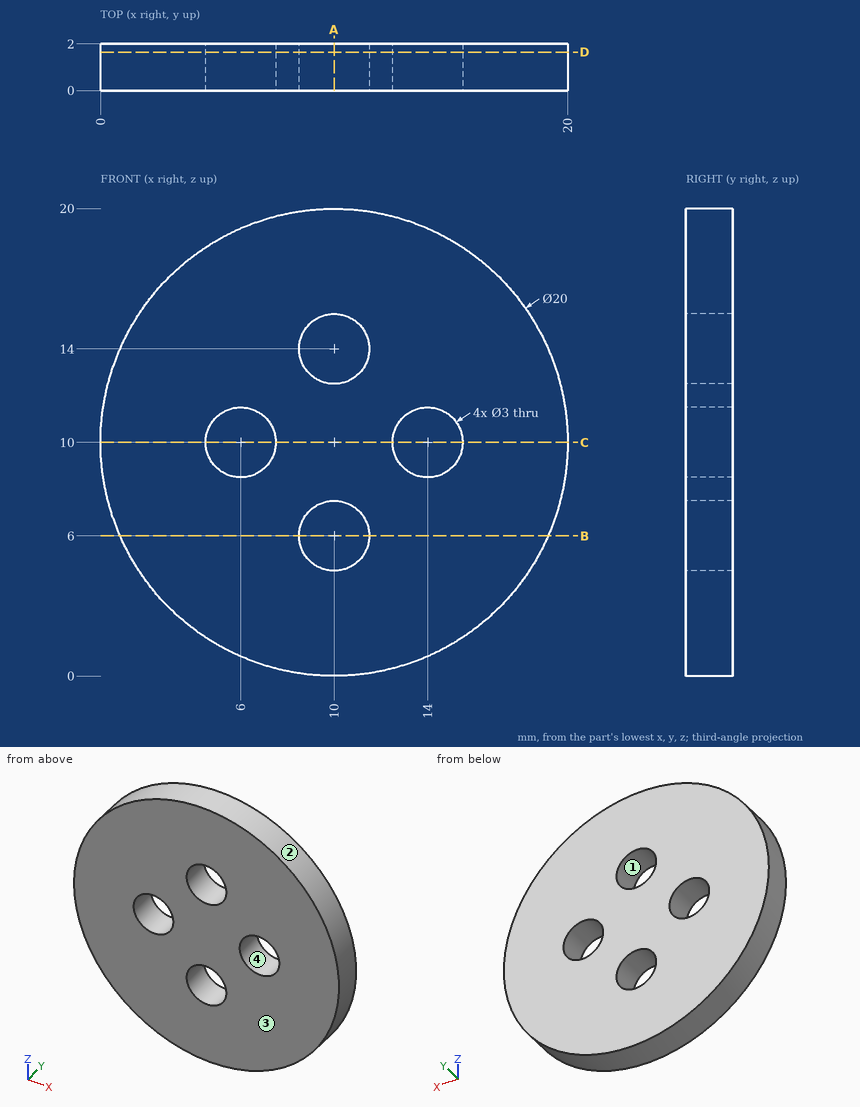
The drawing under review shows one solid part. Ordinate dimensions are in mm from its lowest x, y, z. Round coordinates to 2 decimals unless told otherwise and drop trailing zeros. Write each loop counter-clockwise with the first axis right and the second up, starting at its lowest first coordinate (ties: lowest second). Pieces come first, ordered by that corner, then holes.
(1) Wall thickness on L1, parallel to Z at x = 10, y = 0.8; L2, parallel to X at y = 0.25, z = 10.75; L3, parallel to Z at x = 6, y = 0.8: over which ranges is each line inside the solid? List them lowest first.
(2) We need section C-C on z = 10. Give the boundary of the cut face in (x, y).
(3) Insertion check: pin 1 (1 mm diameter, centred on y = 1.5, z = 4, fed in from -X). The pin has a flat end and moves straight along its axis. Give the tip position at first contact, or say it passes through.
(4) We need section A-A on x = 10. Give the boundary of the cut face in (y, z), and give its area (3 significant figures).
(5) We need section D-D on y = 1.65. Give the boundary of the cut face in (x, z).
(6) Mouldability with a two-part tool opening along X and no side actions: class the marked faces 1, 2, 3 and 4 as +X half, -X half, draft (parallel to the pull), parting line (faces both ways), or undercut.
(7) We need section B-B on z = 6. Give the boundary of the cut face in (x, y).
Findings below:
1. L1: z = 0 to 4.5, 7.5 to 12.5, 15.5 to 20
1. L2: x = 0.03 to 4.7, 7.3 to 12.7, 15.3 to 19.97
1. L3: z = 0.83 to 8.5, 11.5 to 19.17
2. outline: (0, 0) - (4.5, 0) - (4.5, 2) - (0, 2) - close; (7.5, 0) - (12.5, 0) - (12.5, 2) - (7.5, 2) - close; (15.5, 0) - (20, 0) - (20, 2) - (15.5, 2) - close
3. pin 1: stops at x = 1.65
4. outline: (0, 0) - (2, 0) - (2, 4.5) - (0, 4.5) - close; (0, 7.5) - (2, 7.5) - (2, 12.5) - (0, 12.5) - close; (0, 15.5) - (2, 15.5) - (2, 20) - (0, 20) - close
4. area: 28.0 mm2
5. outline: circle Ø20 at (10, 10); hole circle Ø3 at (6, 10); hole circle Ø3 at (10, 6); hole circle Ø3 at (10, 14); hole circle Ø3 at (14, 10)
6. face 1: undercut
6. face 2: parting line
6. face 3: draft
6. face 4: undercut
7. outline: (0.83, 0) - (8.5, 0) - (8.5, 2) - (0.83, 2) - close; (11.5, 0) - (19.17, 0) - (19.17, 2) - (11.5, 2) - close
